from build123d import *

# Parameters (mm, degrees)
F0_W         = 10.2
F0_H         = 2
F1_DEPTH     = 1.5
F2_W         = 12.64
F2_H         = 28.1
F3_DEPTH     = 25
F4_W         = 1.5
F4_H         = 75.9369339572
F5_DEPTH     = 10.5
F6_W         = 35.25
F6_H         = 10.5
F6_R         = 1.3
F6_W_2       = 15.825
F6_W_3       = 9.3619339572
F7_DEPTH     = 25
F9_DEPTH     = 0.5
F10_T1_DEPTH = 18.4
F11_W        = 18.4
F11_H        = 1.5
F11_W_2      = 1.1665335146
F12_DEPTH    = 11.5
F14_DEPTH    = 1.5
F15_DEPTH    = 1.5


# Not quite as in the source:
# - a fillet or chamfer that OpenCascade refuses, or shapes differently, is made with other operations: its cross-section is extruded or revolved along the edge and cut away or added


with BuildPart() as f1:
    # F0 (on Top) → F1 (new body)
    with BuildSketch(Plane.XY):
        Polygon((12.9583973216, 49.6379526287), (-5.4416026784, 49.6379526287), (-5.4416026784, -26.2989813285), (-1.3416026784, -29.5620473713), (8.8583973216, -29.5620473713), (12.9583973216, -26.2989813285), align=None)
        with Locations((3.7583973216, -30.5620473713)):
            Rectangle(F0_W, F0_H)
    extrude(amount=F1_DEPTH)

    # F2 (on face) → F3 (cut)
    with BuildSketch(Plane.XY.offset(1.5)):
        with Locations((4.0783973216, 11.1379526287)):
            Rectangle(F2_W, F2_H)
    extrude(amount=-F3_DEPTH, mode=Mode.SUBTRACT)

    # F4 (on face) → F5 (join)
    with BuildSketch(Plane(origin=(0, 0, 0), x_dir=(1, 0, 0), z_dir=(0, 0, -1))):
        with Locations((-4.6916026784, -11.6694856501)):
            Rectangle(F4_W, F4_H)
    extrude(amount=F5_DEPTH)

    # F6 (on face) → F7 (cut)
    with BuildSketch(Plane.YZ.offset(-3.9416026784)):
        with Locations((8.4379526287, -5.25)):
            Rectangle(F6_W, F6_H)
        with Locations((-13.0620473713, -6.8)):
            Circle(F6_R)
        with Locations((29.9379526287, -6.8)):
            Circle(F6_R)
        with Locations((41.7254526287, -5.25)):
            Rectangle(F6_W_2, F6_H)
        with Locations((-21.6180143499, -5.25)):
            Rectangle(F6_W_3, F6_H)
    extrude(amount=-F7_DEPTH, mode=Mode.SUBTRACT)

    # F8 (on face) → F9 (cut)
    with BuildSketch(Plane(origin=(0, 0, 0), x_dir=(1, 0, 0), z_dir=(0, 0, -1))):
        Polygon((-5.4416026784, 26.2989813285), (-5.4416026784, 23.5620473713), (12.9583973216, 23.5620473713), (12.9583973216, 26.2989813285), (8.8583973216, 29.5620473713), (8.8583973216, 31.5620473713), (-1.3416026784, 31.5620473713), (-1.3416026784, 29.5620473713), align=None)
    extrude(amount=-F9_DEPTH, mode=Mode.SUBTRACT)

    # F10: fillet of radius 5 on 1 edges, made by hand

    # F10_s2 → F10_t1 (join)
    with BuildSketch(Plane.YZ.offset(-5.4416026784)):
        with BuildLine():
            ThreePointArc((-25.7414968431, 0.5), (-24.6234628544, 0.3733971724), (-23.5620473713, 0))
            Line((-23.5620473713, 0), (-23.5620473713, 0.5))
            Line((-23.5620473713, 0.5), (-25.7414968431, 0.5))
        make_face()
    extrude(amount=F10_T1_DEPTH)

    # F11 (on face) → F12 (join)
    with BuildSketch(Plane.XY.offset(1.5)):
        with Locations((3.7583973216, 48.8879526287)):
            Rectangle(F11_W, F11_H)
        with Locations((13.5416640789, 48.8879526287)):
            Rectangle(F11_W_2, F11_H)
    extrude(amount=F12_DEPTH)

    # F13 (on face) → F14 (cut, through all)
    with BuildSketch(Plane(origin=(0, 49.6379526287, 0), x_dir=(-1, 0, 0), z_dir=(0, 1, 0))):
        with BuildLine():
            Line((-12.9583973216, 9.5), (-14.1249308363, 9.5))
            Line((-14.1249308363, 9.5), (-14.1249308363, 5.5))
            Line((-14.1249308363, 5.5), (-12.9583973216, 5.5))
            Line((-12.9583973216, 5.5), (-8.9583973216, 5.5))
            ThreePointArc((-8.9583973216, 5.5), (-10.9583973216, 7.5), (-8.9583973216, 9.5))
            Line((-8.9583973216, 9.5), (-12.9583973216, 9.5))
        make_face()
        with BuildLine():
            ThreePointArc((-6.9583973216, 7.5), (-7.5441837593, 8.9142135624), (-8.9583973216, 9.5))
            ThreePointArc((-8.9583973216, 9.5), (-10.9583973216, 7.5), (-8.9583973216, 5.5))
            ThreePointArc((-8.9583973216, 5.5), (-7.5441837593, 6.0857864376), (-6.9583973216, 7.5))
        make_face()
    extrude(amount=-F14_DEPTH, mode=Mode.SUBTRACT)

    # F15 (add, through all): a face of the model
    f15_faces = [f1.faces().sort_by_distance(p)[0] for p in [
        (13.5416640789, 48.8879526287, 1.5),
    ]]
    extrude(f15_faces, amount=F15_DEPTH)


solid = f1.part
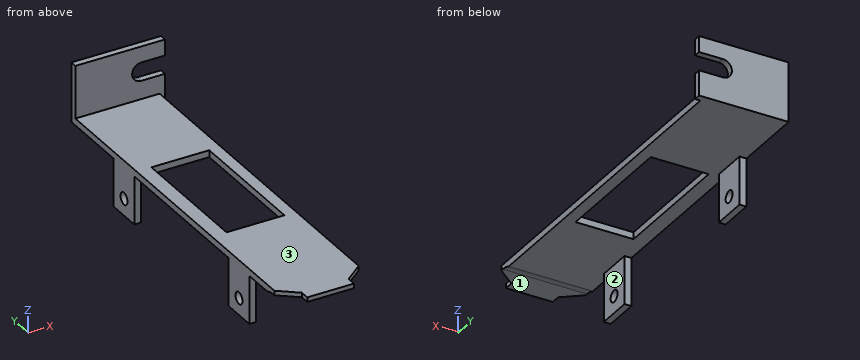
The model under review builds one solid part; all positions refer to its coordinate system, in mm. Face numbers are marked on the shaded views. A direction names the side the tool comes from. Round coordinates to 2 decimals unless told otherwise and drop trailing zeros. Loops run counter-clockwise (first coordinate to the right, second up) from the corner with the lowest first, then second, coordinate; pieces in that order, holes last. Notation, with made-up numbers: (85, 35.5) -> (103, 35.5) arc R25 ccw to (103, 56.5) -> close; hole circle Ø2 at (54.25, 3.25). An arc over 180 degrees is marked (long way). Return JSON: item names as keys, results as strings.
(1) For pin 1 (2 mm diameter, centred on x = -0.5, y = 30, fed in from -Z); pin 2 (12 mm diameter, centred on y = 35, z = 2, fed in from +X); pin 3 (1.6 mm diameter, centred on x = -5, z = -7, fed in from -Y); pin 4 (10 mm diameter, centred on x = 1, z = -1, fed in from +Y), all flat-tipped, find the tip position at first contact; note any pin that passes through.
Solved:
{"pin 1": "z = 0", "pin 2": "x = 12.96", "pin 3": "y = -16.94", "pin 4": "y = 49.64"}
(2) Add section C-C on y = 21. Write out the cut boundary in (x, z), plus the area to 3 significant figures.
Solved:
{"outline": "(-5.44, 0) -> (-2.24, 0) -> (-2.24, 1.5) -> (-5.44, 1.5) -> close; (10.4, 0) -> (12.96, 0) -> (12.96, 1.5) -> (10.4, 1.5) -> close", "area": "8.64 mm2"}
(3) Add section D-D on z = 3.5. Write out the cut boundary in (x, y), plus the area to 3 significant figures.
Solved:
{"outline": "(-5.44, 48.14) -> (14.12, 48.14) -> (14.12, 49.64) -> (-5.44, 49.64) -> close", "area": "29.3 mm2"}
(4) For line 1 (X direction, y = 15.5, z = 0.5); line 2 (Y direction, x = -3, z = 9); line 3 (Z direction, x = 12.75, y = 39), list the stretches that pass through material, from the lowest coordinate up.
Solved:
{"line 1": "-5.44 to -2.24, 10.4 to 12.96", "line 2": "48.14 to 49.64", "line 3": "0 to 1.5"}
(5) For the marked faces 1, 2 and 3, list the 3-axis set-ups (+Z, -Z, +X, -X, +Y, -Y) from which the entire face can be reached by the end or side of a thin tool; tool diameter is ignored.
Solved:
{"face 1": "-Z, +X, -X, -Y", "face 2": "-Z, +X, +Y, -Y", "face 3": "+Z, +X, -X, -Y"}
(6) Add section A-A on z = -4.75. Write out the cut boundary in (x, y).
Solved:
{"outline": "(-5.44, -16.94) -> (-3.94, -16.94) -> (-3.94, -9.19) -> (-5.44, -9.19) -> close; (-5.44, 26.06) -> (-3.94, 26.06) -> (-3.94, 33.81) -> (-5.44, 33.81) -> close"}
(7) Add section B-B on x = 4.75. Write out the cut boundary in (y, z).
Solved:
{"outline": "(-31.56, 0.5) -> (-25.74, 0.5) arc R5 cw to (-23.56, 0) -> (-2.91, 0) -> (-2.91, 1.5) -> (-31.56, 1.5) -> close; (25.19, 0) -> (49.64, 0) -> (49.64, 13) -> (48.14, 13) -> (48.14, 1.5) -> (25.19, 1.5) -> close"}
